Part print with two shaded views. Sizes in mm from the minimum x, y, z corner. A direction names the side the tool comes from. Give positions to 0.01 mm unless a question says otherwise; leave off trailing zeros. Loops run counter-clockwise (first coordinate to the right, second up) from the corner with the lowest first, then second, coordinate; pieces in that order, holes last. Notation, with made-up numbers: M 76.5,1.5 L 105.5,1.5 A18 ccw 105.5,21.5 Z; hole C 86,55 d9. An arc over 180 degrees is marked long. Answer as a JSON object with one key per item and string values. Group by question number.
1. Drop flat-ended pins along their axis: pin 1 Ø4 at (y, z) = (1.5, 10) entering from +X; pin 2 Ø2.5 at (x, y) = (5.5, 6.5) entering from -Z; pin 3 Ø1.5 at (y, z) = (6, 12) entering from -X. Give the stop position or say it passes through.
2. Slice it at D-D (z = 9.5). List the corners of the cut face in (x, y), then the cut area to 3 significant figures.
3. Mould opens along X. For the marked faces 1, 2 and 3 say: released by +X, released by -X, zero draft, split by the parting line, or undercut.
4. 3-axis set-ups, long thin cutter, end or side, ignore diameter. For the marked faces 4, 5 and 6: which of +Z, -Z, +X, -X, +Y, -Y reach the whole face in a straight line?
5. Slice it at C-C (z = 5.75). List the corners of the cut face in (x, y), then the cut area to 3 significant figures.
6. Drill centre lines: line 1 along Y through (x, z) = (6, 6); line 2 along Z through (x, y) = (5.5, 7.25); line 3 along Z through (x, y) = (7.5, 2.5). Where is each one in solid material? Low to high. Write a range as [from, to].
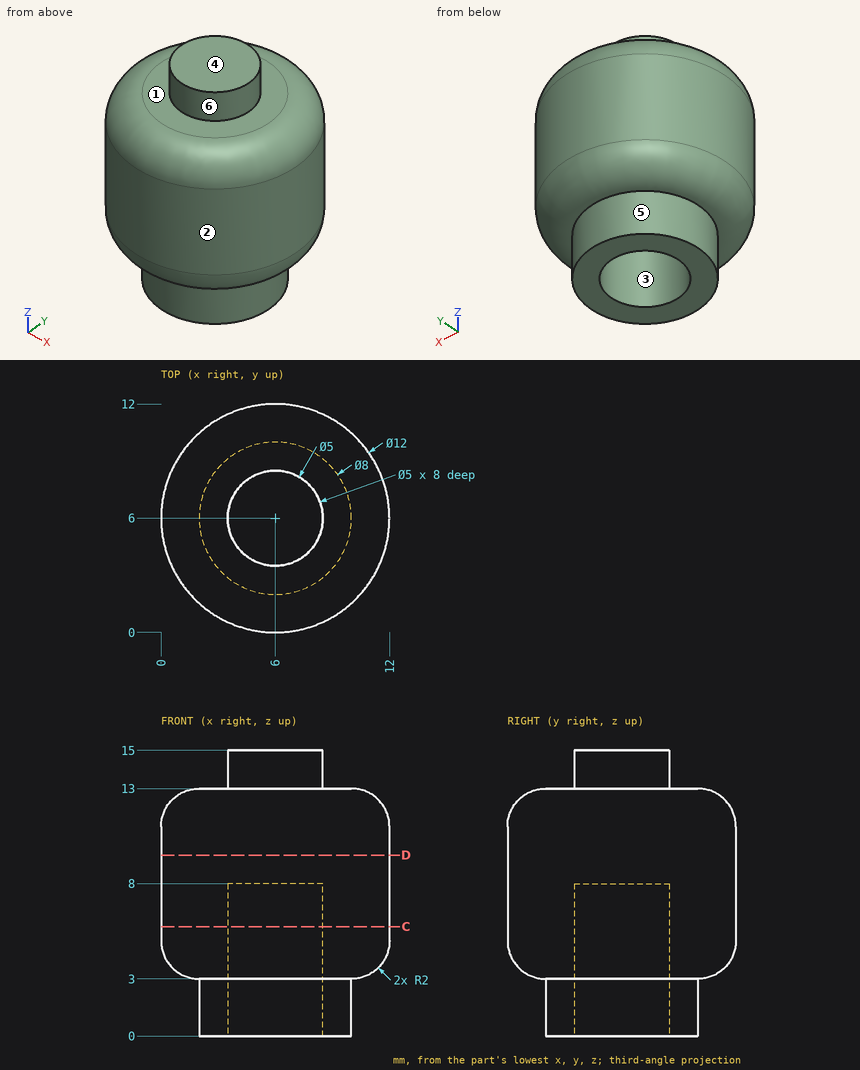
Established:
{
 "1": {"pin 1": "stops at x = 11.45", "pin 2": "stops at z = 8", "pin 3": "stops at x = 0.02"},
 "2": {"outline": "C 6,6 d12", "area": "113 mm^2"},
 "3": {"face 1": "zero draft", "face 2": "split by the parting line", "face 3": "undercut"},
 "4": {"face 4": "+Z, +X, -X, +Y, -Y", "face 5": "-Z", "face 6": "+Z"},
 "5": {"outline": "C 6,6 d12; hole C 6,6 d5", "area": "93.5 mm^2"},
 "6": {"line 1": "y = [0, 3.5], [8.5, 12]", "line 2": "z = [8, 15]", "line 3": "z = [0, 13]"}
}
